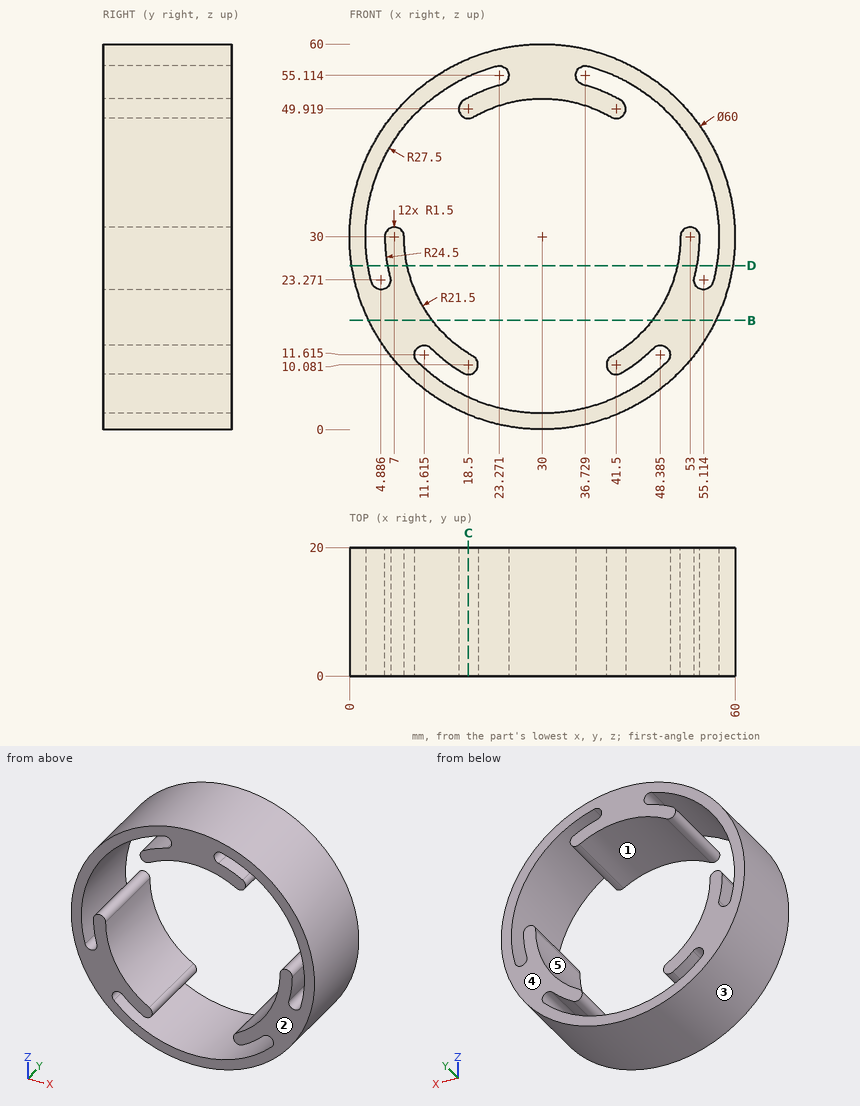
Geometry check sheet. Reference: drawing and pictorial views, mm from the part's lowest x, y, z. A direction names the side the tool comes from. Coordinates: 2 decimals unless noted, no trailing zeros. Order: outer loops, then holes, each group sorted by start corner. A loop starts at its lowest first (then second) coordinate and runs counter-clockwise, first axis right, second up. Notation, with made-up numbers: (35, -27) -> (53, -27) arc R11 ccw to (53, -18) -> close; hole circle Ø5 at (43, 38.25). An arc over 180 degrees is marked (long way). Write item = value, one per line. Start each with the question number.
1) Access from +Z, -Z, +X, -X, +Y, -Y to the whole of each face (thin tool, end or side, straight path). Record for the marked faces 4 and 5.
2) Cross-section at D-D (z = 25.5). Enter the section's corners in (x, y).
3) Go/stop test with flat-tipped pins: P1, Ø10, axis at x = 46.5, z = 31.5, coming from the -Y side; P2, Ø5, axis at y = 4, z = 44, coming from the -X side; P3, Ø10, axis at y = 2, z = 53.5, coming from the +X side; P4, Ø1.5, axis at x = 22, y = 18, coming from the -Z side. Record where each tip stops, or that it passes through.
4) Cross-section at B-B (z = 17). Enter the section's corners in (x, y) (1 decimal).
5) Cross-section at C-C (x = 18.5). Enter the section's corners in (y, z).
6) Material ranges on L1, parallel to Z at x = 49, y = 17.5 (1 decimal); L2, parallel to Z at x = 30.5, y = 14.75 (1 decimal); L3, parallel to X at y = 4, z = 26 (1 decimal), recorded low to high.
7) Mould release check, pull along Z, two halves, no side actions. Record for the marked faces 1, 2 and 3: +Z half, -Z half, draft (parallel to the pull), parting line (faces both ways), or undercut.
Ans:
q1.face_4 = +Z, -Z, +X, -X, +Y
q1.face_5 = +Y, -Y
q2.outline = (0.34, 0) -> (2.87, 0) -> (2.87, 20) -> (0.34, 20) -> close; (5.92, 0) -> (8.98, 0) -> (8.98, 20) -> (5.92, 20) -> close; (51.02, 0) -> (54.08, 0) -> (54.08, 20) -> (51.02, 20) -> close; (57.13, 0) -> (59.66, 0) -> (59.66, 20) -> (57.13, 20) -> close
q3.P1 = through
q3.P2 = 2.29
q3.P3 = 53.62
q3.P4 = 0.89
q4.outline = (3, 0) -> (12.9, 0) -> (12.9, 20) -> (3, 20) -> close; (47.1, 0) -> (57, 0) -> (57, 20) -> (47.1, 20) -> close
q5.outline = (0, 2.29) -> (20, 2.29) -> (20, 5.02) -> (0, 5.02) -> close; (0, 8.58) -> (20, 8.58) -> (20, 11.83) -> (0, 11.83) -> close; (0, 48.42) -> (20, 48.42) -> (20, 51.63) -> (0, 51.63) -> close; (0, 54.98) -> (20, 54.98) -> (20, 57.71) -> (0, 57.71) -> close
q6.L1 = 6.8 to 10.1, 13 to 19.9, 49.9 to 53.2
q6.L2 = 0 to 2.5, 51.5 to 60
q6.L3 = 0.3 to 2.8, 5.8 to 8.9, 51.1 to 54.2, 57.2 to 59.7
q7.face_1 = undercut
q7.face_2 = draft
q7.face_3 = parting line
